from build123d import *


with BuildPart() as part:
    # Sketch2 → Revolve1 (revolve)
    with BuildSketch(Plane.XY, mode=Mode.PRIVATE) as revolve1_sk:
        with BuildLine():
            Line((38.1, 7.9375), (34.925, 7.9375))
            Line((34.925, 7.9375), (34.925, 12.7))
            Line((34.925, 12.7), (0, 12.7))
            Line((0, 12.7), (0, 0))
            Line((0, 0), (0, -44.45))
            ThreePointArc((0, -44.45), (25.664225243, -32.512774616), (33.069273235, -5.194006865))
            ThreePointArc((33.069273235, -5.194006865), (39.309985781, -4.181816741), (42.036043974, 1.52253499))
            ThreePointArc((42.036043974, 1.52253499), (44.580012514, 7.310388306), (41.275, 12.7))
            Line((41.275, 12.7), (38.1, 12.7))
            Line((38.1, 12.7), (38.1, 7.9375))
        make_face()
    revolve(revolve1_sk.sketch.rotate(Axis((0, 12.7, 0), (0, -1, 0)), 180), axis=Axis((0, 12.7, 0), (0, -1, 0)))


solid = part.part
For this review, take the finished solid that the model builds, in its own axes (mm). A direction names the side the tool comes from. Round coordinates to 2 decimals unless told otherwise and drop trailing zeros. Order: outer loops, then holes, each group sorted by start corner. A loop starts at its lowest first (then second) coordinate and runs counter-clockwise, first axis right, second up. Notation, with made-up numbers: M 47,-11.5 L 80,-11.5 A17 cw 80,10.5 Z; hole C 6,16.25 d7. An arc over 180 degrees is marked long. Write each question's results on one line, items separated by ' | '. Start each with the question number.
1. To check wall thickness, follow L1, parallel to Z at x = 0, y = 10.95 (3 decimals); L2, parallel to Z at x = 0, y = 10 (3 decimals); L3, parallel to X at y = 9.5, z = -21. State the ranges of each line that lie inside material, in increasing order. Write a range as [from, to].
2. Add section B-B (x = 0). State the section outline as (y, z) points (1 decimal), then the cut area to 3 significant figures.
3. Draft analysis for pull direction X (two halves, no side actions). For faces 3 (the face through (0, 12.7, 0)), 4 (the face through (7.571, 10.352, 34.094)), state which applies: pulls with the +X half, pulls with the -X half, needs draft (parallel to the pull), parting line crosses it, or undercut.
4. Clearance check with flat-ended pins moving along their axes: pin 1 Ø1 at (x, y) = (-20, -19) entering from +Z; pin 2 Ø4 at (x, y) = (21, -30.5) entering from +Z; pin 3 Ø6 at (x, y) = (8, -36) entering from +Z. State where each tip first meets the part, or that it passes through.
5. Tool access review of faces 1 (the face through (-17, 7.938, 31)), 2 (the face through (-12, 12.7, 36.5)): name each direction out of +Z, -Z, +X, -X, +Y, -Y from which nothing blocks a thin tool from reaching the whole face with its end or side.
6. Add section C-C (y = -12). State the section outline as (x, z) points.
Output values:
1) L1: [-43.223, -38.1], [-34.925, 34.925], [38.1, 43.223] | L2: [-43.823, -38.1], [-34.925, 34.925], [38.1, 43.823] | L3: [-38.73, -31.79], [-27.91, 27.91], [31.79, 38.73]
2) outline: M -5.2,-33.1 A6.8 ccw 1.5,-42 A6.8 ccw 12.7,-41.3 L 12.7,-38.1 L 7.9,-38.1 L 7.9,-34.9 L 12.7,-34.9 L 12.7,34.9 L 7.9,34.9 L 7.9,38.1 L 12.7,38.1 L 12.7,41.3 A6.8 ccw 1.5,42 A6.8 ccw -5.2,33.1 A33.6 ccw long Z | area: 3,650 mm^2
3) face 3: needs draft | face 4: undercut
4) pin 1: z = 26.11 | pin 2: z = 20.29 | pin 3: z = 24.1
5) face 1: +Y | face 2: +Z, -Z, +X, -X, +Y
6) outline: C 0,0 d67.08
